The model under review builds one solid part; all positions refer to its coordinate system, in mm. A direction names the side the tool comes from. Round coordinates to 2 decimals unless told otherwise and drop trailing zeros. Order: outer loops, then holes, each group sorted by start corner. A loop starts at its lowest first (then second) coordinate and runs counter-clockwise, first axis right, second up.
1) Machinability: for faces 5 (the face through (-1, -1, -52)), 6 (the face through (0, -7, -47)), which of the approach directions +Z, -Z, +X, -X, +Y, -Y give a long, thin tool a straight path to every point of the face, cutting with its end or side? Answer none if there is none.
2) Consider section D-D (y = -5.75). Give the boundary of the cut face in (x, z).
3) To check wall thickness, follow L1, parallel to X at y = -2, z = -32; L2, parallel to Z at x = 1, y = -2.25; L3, parallel to X at y = -1, z = -48.75. State the ranges of each line that lie inside material, in increasing order.
4) Clearance check with flat-ended pins moving along their axes: P1, Ø5, axis at x = 18, y = -4, coming from the -Z side; P2, Ø1.5, axis at x = 15.5, y = -5.5, coming from the -Z side; P3, Ø4, axis at y = -2.5, z = -47.5, coming from the -X side. State where each tip first meets the part, or that it passes through.
5) Consider section B-B (z = -42.5). Give the boundary of the cut face in (x, y).
6) Consider section A-A (x = 23.5). Give the boundary of the cut face in (y, z).
7) Mouldability with a two-part tool opening along Z and no side actions: class faces 1 (the face through (37.9, -3.55, -27.73)), 2 (the face through (0, -2, -52)), 3 (the face through (1, -1, -52)), 4 (the face through (-3.6, 2, -56.2)) as pulls with the +Z half, pulls with the -Z half, needs draft (parallel to the pull), parting line crosses it, or undercut.
8) Consider section C-C (z = -51.75). Give the boundary of the cut face in (x, y), then the cut area to 3 significant figures.
from build123d import *

# Parameters (mm, degrees)
BOSS_EXTRUDE1_DEPTH = 7
SKETCH2_W           = 2
SKETCH2_H           = 9.756485423
BOSS_EXTRUDE2_DEPTH = 2
BOSS_EXTRUDE3_DEPTH = 2
FILLET1_R           = 0.5
FILLET2_R           = 1.5


with BuildPart() as part:
    # Sketch1 → Boss-Extrude1 (new body)
    with BuildSketch(Plane(origin=(0, 0, 0), x_dir=(1, 0, 0), z_dir=(0, 1, 0))):
        with BuildLine():
            Line((37.784873439, 27.102644506), (46.515434438, 33.801839581))
            ThreePointArc((46.515434438, 33.801839581), (0, 57.5), (-46.515434438, 33.801839581))
            Line((-46.515434438, 33.801839581), (-37.784873439, 27.102644506))
            ThreePointArc((-37.784873439, 27.102644506), (0, 46.5), (37.784873439, 27.102644506))
        make_face()
        with BuildLine():
            Line((-38.080960334, 29.220548592), (-44.427787056, 34.090640024))
            ThreePointArc((-44.427787056, 34.090640024), (0, 56), (44.427787056, 34.090640024))
            Line((44.427787056, 34.090640024), (38.080960334, 29.220548592))
            ThreePointArc((38.080960334, 29.220548592), (0, 48), (-38.080960334, 29.220548592))
        make_face(mode=Mode.SUBTRACT)
    extrude(amount=-BOSS_EXTRUDE1_DEPTH)

    # Sketch2 → Boss-Extrude2 (add)
    with BuildSketch(Plane(origin=(0, 0, 0), x_dir=(1, 0, 0), z_dir=(0, 1, 0))):
        with Locations((0, 51.881238044)):
            Rectangle(SKETCH2_W, SKETCH2_H)
    extrude(amount=-BOSS_EXTRUDE2_DEPTH)

    # Sketch3 → Boss-Extrude3 (add)
    with BuildSketch(Plane(origin=(0, 0, 0), x_dir=(1, 0, 0), z_dir=(0, 1, 0))):
        with BuildLine():
            Line((45.324988438, 32.888378237), (46.515434438, 33.801839581))
            ThreePointArc((46.515434438, 33.801839581), (0, 57.5), (-46.515434438, 33.801839581))
            Line((-46.515434438, 33.801839581), (-45.324988438, 32.888378237))
            ThreePointArc((-45.324988438, 32.888378237), (0, 56), (45.324988438, 32.888378237))
        make_face()
    extrude(amount=BOSS_EXTRUDE3_DEPTH)

    # Fillet1
    fillet1_edges = [part.edges().sort_by_distance(p)[0] for p in [
        (-38.080960334, -3.5, -29.220548592),
        (-44.427787056, -3.5, -34.090640024),
        (38.080960334, -3.5, -29.220548592),
        (44.427787056, -3.5, -34.090640024),
    ]]
    fillet(fillet1_edges, radius=FILLET1_R)

    # Fillet2
    fillet2_edges = [part.edges().sort_by_distance(p)[0] for p in [
        (46.515434438, -2.5, -33.801839581),
        (37.784873439, -3.5, -27.102644506),
        (-37.784873439, -3.5, -27.102644506),
        (-46.515434438, -2.5, -33.801839581),
    ]]
    fillet(fillet2_edges, radius=FILLET2_R)


solid = part.part
Answer below:
1. face 5: +Y, -Y
1. face 6: +Z, -Z, +X, -X, -Y
2. outline: (-45.62, -35) arc R57.5 ccw to (45.62, -35) arc R1.5 ccw to (45.34, -32.9) - (38.99, -28.03) arc R1.5 ccw to (36.89, -28.31) arc R46.5 cw to (-36.89, -28.31) arc R1.5 ccw to (-38.99, -28.03) - (-45.34, -32.9) arc R1.5 ccw to start; hole (-44.12, -34.49) arc R56 ccw to (44.12, -34.49) arc R0.5 ccw to (44.03, -33.78) - (38.48, -29.52) arc R0.5 ccw to (37.78, -29.61) arc R48 cw to (-37.78, -29.61) arc R0.5 ccw to (-38.48, -29.52) - (-44.03, -33.78) arc R0.5 ccw to start
3. L1: x = -44.17 to -41.7, -35.78 to -33.74, 33.74 to 35.78, 41.7 to 44.17
3. L2: z = -57.49 to -55.99, -47.99 to -46.49
3. L3: x = -30.49 to -27.56, -1 to 1, 27.56 to 30.49
4. P1: stops at z = -55.37
4. P2: stops at z = -55.58
4. P3: stops at x = -35.16
5. outline: (-38.73, -7) - (-36.47, -7) - (-36.47, 2) - (-38.73, 2) - close; (-22.31, -7) - (-18.87, -7) - (-18.87, 0) - (-22.31, 0) - close; (18.87, -7) - (22.31, -7) - (22.31, 0) - (18.87, 0) - close; (36.47, -7) - (38.73, -7) - (38.73, 2) - (36.47, 2) - close
6. outline: (-7, -52.48) - (2, -52.48) - (2, -50.83) - (-7, -50.83) - close; (-7, -41.85) - (0, -41.85) - (0, -40.12) - (-7, -40.12) - close
7. face 1: pulls with the +Z half
7. face 2: undercut
7. face 3: undercut
7. face 4: needs draft
8. outline: (-25.06, -7) - (-21.4, -7) - (-21.4, 2) - (-25.06, 2) - close; (-1, -2) - (1, -2) - (1, 0) - (-1, 0) - close; (21.4, -7) - (25.06, -7) - (25.06, 2) - (21.4, 2) - close
8. area: 70.0 mm2
